Source: CAD feature listing. Evaluate the final solid. Frame: model axes, mm. Face numbers are marked on the shaded views. A direction names the side the tool comes from. Give positions to 0.01 mm unless a question says otherwise; leave off trailing zeros. Loops run counter-clockwise (first coordinate to the right, second up) from the corner with the lowest first, then second, coordinate; pieces in that order, holes last. Notation, with made-up numbers: (25.5, 54.5) -> (43.5, 54.5) arc R5 ccw to (43.5, 59.5) -> close; hole circle Ø1 at (17.5, -25.75). An arc over 180 degrees is marked (long way). Return JSON: item names as keys, results as strings. Group by question number.
(1) Access query for the marked faces 4, 5, 6 and 7. Directions: +Z, -Z, +X, -X, +Y, -Y. A direction counts if a zero-diameter tool reaches every point of the face in a straight line with its end or side. Return the directions, or none.
(2) Ray query, line 1 (Y direction, x = -11.5, z = 15); line 2 (X direction, y = -3.5, z = -8); line 3 (X direction, y = -21.5, z = 11). Return the intervals inside material, ascending. Write a range as from..to.
(3) Cut plane A-A on y = -45.5. Return loops of the section in (x, z).
(4) Cut plane B-B on z = -7. Return loops of the section in (x, y).
(5) Cut plane C-C on y = -39. Return loops of the section in (x, z).
(6) Pin query (flat end, axial travel): pin 1 (3 mm diameter, centred on x = -0.5, z = 12.5, fed in from +Y); pin 2 (5 mm diameter, centred on y = -7.5, z = -5.5, fed in from -X); pin 3 (1.9 mm diameter, centred on x = 89, y = -37.5, fed in from -Z); pin 4 (9.5 mm diameter, centred on x = 77.5, z = -7, fed in from +Y). Return the tip coordinate at first contact, or that it passes through.
(7) Draft query along X for the marked faces 1, 2 and 3. Return one class per face: released by +X, released by -X, zero draft, split by the parting line, or undercut.
(8) Cut plane D-D on x = 57.5. Return loops of the section in (y, z), then the cut area to 3 significant figures.
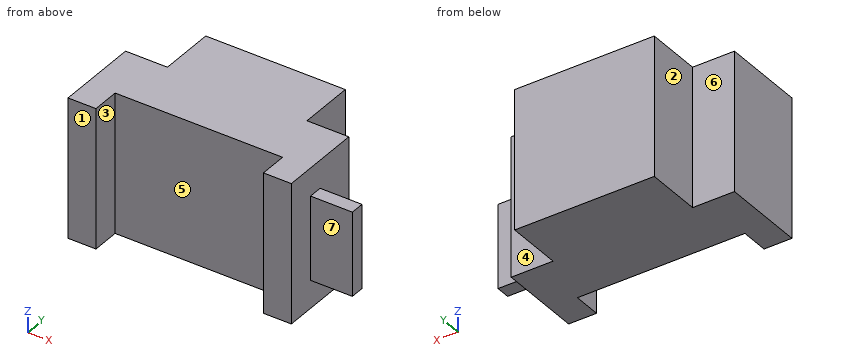
Autodesk Inventor part; units mm, degrees
ref_plane "YZ Plane" through (0, 0, 0) normal (1, 0, 0) x (0, 1, 0)
ref_plane "XZ Plane" through (0, 0, 0) normal (0, 1, 0) x (-1, 0, 0)
ref_plane "XY Plane" through (0, 0, 0) normal (0, 0, 1) x (1, 0, 0)
sketch "Sketch1" plane through (0, 0, 0) normal (1, 0, 0) x (0, 1, 0)
  line L0 (9.5985, 34.7638) -> (-15.8015, 34.7638)
  line L1 (-15.8015, 34.7638) -> (-15.8015, -28.7362)
  line L2 (-15.8015, -28.7362) -> (9.5985, -28.7362)
  line L3 (9.5985, -28.7362) -> (9.5985, 34.7638)
  point P0 (0, 0)
  dimension "d0" = 25.4
  dimension "d1" = 63.5
extrude "Extrusion1" add sketch "Sketch1" along normal blind 63.5
sketch "Sketch2" plane through (0, -15.8015, 34.7638) normal (0, 0, 1) x (1, 0, 0)
  line L0 (0, 0) -> (63.5, 0)
  line L1 (31.75, 0) -> (-19.05, 0)
  line L2 (-19.05, 0) -> (82.55, 0)
  line L3 (82.55, 0) -> (82.55, -25.4)
  line L4 (82.55, -25.4) -> (-19.05, -25.4)
  line L5 (-19.05, -25.4) -> (-19.05, 0)
  point P0 (0, 15.8015)
  dimension "d4" = 50.8
  dimension "d5" = 101.6
  dimension "d6" = 25.4
extrude "Extrusion2" add sketch "Sketch2" against normal blind 63.5
sketch "Sketch3" plane through (0, 9.5985, 34.7638) normal (0, 0, 1) x (1, 0, 0)
  line L0 (82.55, -50.8) -> (-19.05, -50.8)
  line L1 (-19.05, -50.8) -> (-19.05, -63.5)
  line L2 (-19.05, -63.5) -> (-6.35, -63.5)
  line L3 (-6.35, -63.5) -> (-6.35, -50.8)
  line L4 (82.55, -50.8) -> (82.55, -63.5)
  line L5 (82.55, -63.5) -> (69.85, -63.5)
  line L6 (69.85, -63.5) -> (69.85, -50.8)
  point P0 (0, -9.5985)
  dimension "d9" = 12.7
  dimension "d10" = 12.7
  dimension "d11" = 12.7
  dimension "d12" = 12.7
extrude "Extrusion3" add sketch "Sketch3" against normal blind 63.5
sketch "Sketch4" plane through (82.55, -15.8015, 34.7638) normal (1, 0, 0) x (0, 0, -1)
  line L0 (0, 0) -> (63.5, 0)
  line L1 (31.75, -19.05) -> (12.7, -19.05)
  line L2 (12.7, -19.05) -> (50.8, -19.05)
  line L3 (50.8, -19.05) -> (50.8, -25.4)
  line L4 (0, -25.4) -> (63.5, -25.4)
  line L5 (50.8, -25.4) -> (12.7, -25.4)
  line L6 (12.7, -25.4) -> (12.7, -19.05)
  point P0 (34.7638, 15.8015)
  dimension "d16" = 19.05
  dimension "d17" = 38.1
  dimension "d18" = 6.35
  dimension "d19" = 38.1
  dimension "d20" = 6.35
extrude "Extrusion4" add sketch "Sketch4" along normal blind 19.05
Answers:
{
 "1": {"face 4": "+Z, -Z, +X, +Y", "face 5": "+Z, -Z, -Y", "face 6": "+Z, -Z, -X, +Y", "face 7": "+Z, -Z, +X, -Y"},
 "2": {"line 1": "-53.9..-15.8", "line 2": "0..63.5", "line 3": "-19.05..82.55"},
 "3": {"outline": "(-19.05, -28.74) -> (-6.35, -28.74) -> (-6.35, 34.76) -> (-19.05, 34.76) -> close; (69.85, -28.74) -> (82.55, -28.74) -> (82.55, 34.76) -> (69.85, 34.76) -> close"},
 "4": {"outline": "(-19.05, -53.9) -> (-6.35, -53.9) -> (-6.35, -41.2) -> (69.85, -41.2) -> (69.85, -53.9) -> (82.55, -53.9) -> (82.55, -41.2) -> (101.6, -41.2) -> (101.6, -34.85) -> (82.55, -34.85) -> (82.55, -15.8) -> (63.5, -15.8) -> (63.5, 9.6) -> (0, 9.6) -> (0, -15.8) -> (-19.05, -15.8) -> close"},
 "5": {"outline": "(-19.05, -28.74) -> (82.55, -28.74) -> (82.55, -16.04) -> (101.6, -16.04) -> (101.6, 22.06) -> (82.55, 22.06) -> (82.55, 34.76) -> (-19.05, 34.76) -> close"},
 "6": {"pin 1": "y = 9.6", "pin 2": "x = 0", "pin 3": "z = -16.04", "pin 4": "y = -15.8"},
 "7": {"face 1": "zero draft", "face 2": "released by -X", "face 3": "undercut"},
 "8": {"outline": "(-41.2, -28.74) -> (9.6, -28.74) -> (9.6, 34.76) -> (-41.2, 34.76) -> close", "area": "3,230 mm²"}
}
